from build123d import *

# Parameters (mm, degrees)
F1_DEPTH = 10.16
F2_D     = 3.175
F3_D     = 3.175
F4_D     = 3.175


with BuildPart() as f1:
    # F0 (on Top) → F1 (new body)
    with BuildSketch(Plane.XY):
        Polygon((28.5605379663, 36.279651515), (-29.6971968522, 36.279651515), (-29.6971968522, 0), (-22.248769179, 0), (-22.248769179, -8.4145991132), (-29.6971968522, -8.4145991132), (-29.6971968522, -42.2337416008), (28.5605379663, -42.2337416008), (28.5605379663, -8.4145991132), (21.1078077555, -8.4145991132), (21.1078077555, 0), (28.5605379663, 0), align=None)
    extrude(amount=F1_DEPTH)

    # F2 (through all)
    with Locations(Plane(origin=(0, 0, 0), x_dir=(1, 0, 0), z_dir=(0, 0, -1))):
        with Locations((0, -10.9305603428)):
            Hole(F2_D / 2)

    # F3 (through all)
    with Locations(Plane(origin=(0, 0, 0), x_dir=(1, 0, 0), z_dir=(0, 0, -1))):
        with Locations((0, 19.5694396572)):
            Hole(F3_D / 2)

    # F4 (through all)
    with Locations(Plane(origin=(0, 0, 0), x_dir=(1, 0, 0), z_dir=(0, 0, -1))):
        with Locations((0, 34.5694396572)):
            Hole(F4_D / 2)


solid = f1.part
Work out the finished part from the listing and answer in its coordinate system (mm). A direction names the side the tool comes from. Coordinates: 2 decimals unless noted, no trailing zeros. Write each loop counter-clockwise with the first axis right and the second up, starting at its lowest first coordinate (ties: lowest second). Pieces come first, ordered by that corner, then holes.
1. The part is cut by section B-B, the plane z = 2.25. Write down the section's boundary in (x, y) (1 decimal).
Results list:
outline: (-29.7, -42.2) - (28.6, -42.2) - (28.6, -8.4) - (21.1, -8.4) - (21.1, 0) - (28.6, 0) - (28.6, 36.3) - (-29.7, 36.3) - (-29.7, 0) - (-22.2, 0) - (-22.2, -8.4) - (-29.7, -8.4) - close; hole circle Ø3.2 at (0, -34.6); hole circle Ø3.2 at (0, -19.6); hole circle Ø3.2 at (0, 10.9)
2. For faces 1 (the flat face through (0, 36.28, 5)), 2 (the flat face through (-26, 0, 5)), 3 (the flat face through (25, -8.415, 5)), determine the directions among +Z, -Z, +X, -X, +Y, -Y from which every point of the face is accessible in a straight line to the end or side of a thin tool.
Results list:
face 1: +Z, -Z, +X, -X, +Y
face 2: +Z, -Z, -X
face 3: +Z, -Z, +X
3. Consider line 1 along Y through (x, z) = (0, 3.75); line 2 along Y through (x, z) = (-24, 8.25); line 3 along X through (y, z) = (-4, 0.75). Determine where each line is inside the solid, lowest interval first.
Results list:
line 1: y = -42.23 to -36.16, -32.98 to -21.16, -17.98 to 9.34, 12.52 to 36.28
line 2: y = -42.23 to -8.41, 0 to 36.28
line 3: x = -22.25 to 21.11
4. The part is cut by section A-A, the plane x = 0. Write down the section's boundary in (y, z).
Results list:
outline: (-42.23, 0) - (-36.16, 0) - (-36.16, 10.16) - (-42.23, 10.16) - close; (-32.98, 0) - (-21.16, 0) - (-21.16, 10.16) - (-32.98, 10.16) - close; (-17.98, 0) - (9.34, 0) - (9.34, 10.16) - (-17.98, 10.16) - close; (12.52, 0) - (36.28, 0) - (36.28, 10.16) - (12.52, 10.16) - close
5. The part is cut by section C-C, the plane y = -1. Write down the section's boundary in (x, z), and give its area (3 significant figures).
Results list:
outline: (-22.25, 0) - (21.11, 0) - (21.11, 10.16) - (-22.25, 10.16) - close
area: 441 mm2
6. Flat-ended cylindrical pins translate along their axes: pin 1 (3 mm diameter, centred on x = 16, y = -10, fed in from -Z); pin 2 (4 mm diameter, centred on y = -3.5, z = 3, fed in from +X); pin 3 (4 mm diameter, centred on y = -6, z = 6, fed in from -X); pin 4 (1.9 mm diameter, centred on x = 0, y = 10.93, fed in from -Z). Find the tip coordinate at first contact, or state that the pin passes through.
Results list:
pin 1: stops at z = 0
pin 2: stops at x = 21.11
pin 3: stops at x = -22.25
pin 4: passes through
7. For a pull along X with two mould halves and no side action, classify faces 4 (the cylindrical face through (-0.73, 12.34, 5.15)), 5 (the flat face through (-29.697, -25, 5)), 6 (the flat face through (21.108, -4, 5)), 7 (the flat face through (-1, -2, 0)) as +X half, -X half, draft (parallel to the pull), parting line (faces both ways), or undercut.
Results list:
face 4: undercut
face 5: -X half
face 6: +X half
face 7: draft
